Drawing for the job (mm, zero at the part's lowest x, y, z). A direction names the side the tool comes from. Give positions to 0.01 mm unless a question says otherwise; leave off trailing zeros. Loops run counter-clockwise (first coordinate to the right, second up) from the corner with the lowest first, then second, coordinate; pieces in that order, holes last.
1) Band-saw the part on B-B on y = 3. List the corners of the cut face in (x, z).
2) 3-axis set-ups, long thin cutter, end or side, ignore diameter. For the marked faces 4 and 5: which of +Z, -Z, +X, -X, +Y, -Y reach the whole face in a straight line?
3) Band-saw the part on D-D on x = 11.5. List the corners of the cut face in (y, z) (1 decimal), then the cut area to 3 significant figures.
4) Band-saw the part on A-A on x = 13.5. List the corners of the cut face in (y, z) (1 decimal).
5) Band-saw the part on C-C on y = 9.75. List the corners of the cut face in (x, z) (1 decimal).
6) Flat gauge pins, fed straight in: P1, Ø4, axis at y = 2, z = 9, coming from the +X side; P2, Ø2, axis at x = 12.5, z = 4, coming from the +Y side (1 decimal). Where does each tip first touch, or does it go through?
7) Two-plate mould, pull along X, no slides. Class the marked faces 1, 2 and 3: +X half, -X half, draft (parallel to the pull), parting line (faces both ways), or undercut.
8) Wall check: line 1 (Z direction, x = 12.5, y = 10.5); line 2 (Y direction, x = 8, z = 7) (1 decimal); line 3 (Y direction, x = 8.75, z = 9.5). Give the ranges that are in metal, low to high.
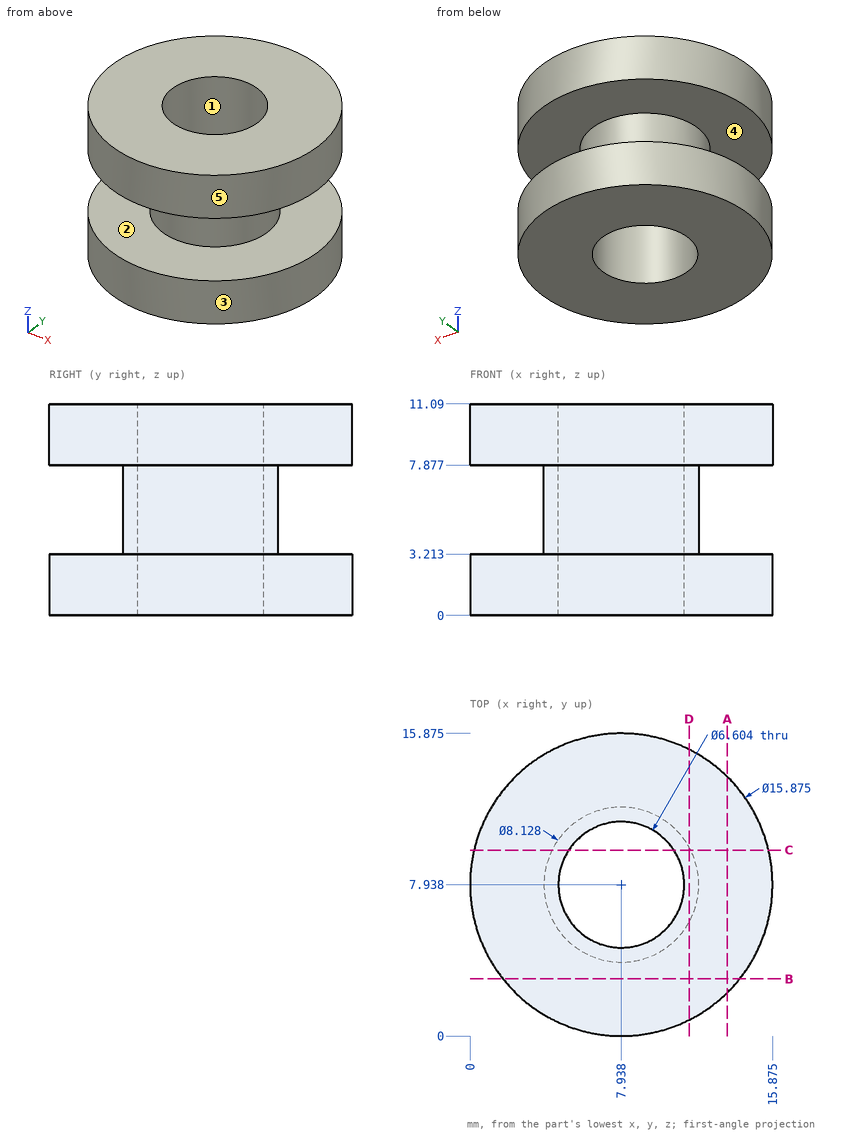
Findings below:
1. outline: (1.72, 0) - (14.15, 0) - (14.15, 3.21) - (1.72, 3.21) - close; (1.72, 7.88) - (14.15, 7.88) - (14.15, 11.09) - (1.72, 11.09) - close
2. face 4: none
2. face 5: +Z, -Z
3. outline: (0.8, 0) - (15, 0) - (15, 3.2) - (9.9, 3.2) - (9.9, 7.9) - (15, 7.9) - (15, 11.1) - (0.8, 11.1) - (0.8, 7.9) - (6, 7.9) - (6, 3.2) - (0.8, 3.2) - close
3. area: 109 mm2
4. outline: (2.3, 0) - (13.6, 0) - (13.6, 3.2) - (2.3, 3.2) - close; (2.3, 7.9) - (13.6, 7.9) - (13.6, 11.1) - (2.3, 11.1) - close
5. outline: (0.2, 0) - (5.2, 0) - (5.2, 11.1) - (0.2, 11.1) - (0.2, 7.9) - (4.3, 7.9) - (4.3, 3.2) - (0.2, 3.2) - close; (10.7, 0) - (15.7, 0) - (15.7, 3.2) - (11.6, 3.2) - (11.6, 7.9) - (15.7, 7.9) - (15.7, 11.1) - (10.7, 11.1) - close
6. P1: stops at x = 14.83
6. P2: stops at y = 14.8
7. face 1: undercut
7. face 2: draft
7. face 3: parting line
8. line 1: z = 0 to 3.21, 7.88 to 11.09
8. line 2: y = 3.9 to 4.6, 11.2 to 12
8. line 3: y = 0.04 to 4.74, 11.14 to 15.83
